Print and shaded views of the part. All mm, measured from the part's lowest x, y and z. A direction names the side the tool comes from. Coordinates: 2 decimals unless noted, no trailing zeros. Order: outer loops, then holes, each group sorted by start corner. A loop starts at its lowest first (then second) coordinate and runs counter-clockwise, first axis right, second up.
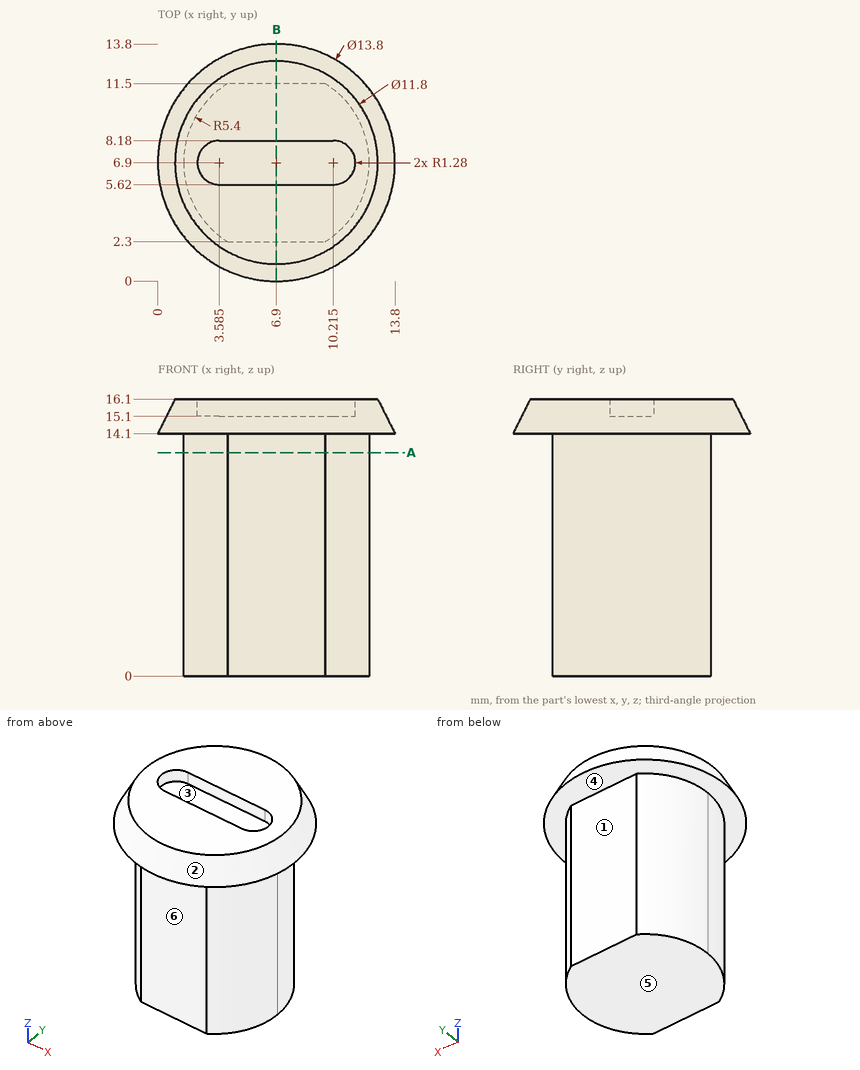
Q1. Drop flat-ended pins along their axis: P1, Ø6, axis at y = 11, z = 10.5, coming from the +X side; P2, Ø1.5, axis at x = 7, z = 3, coming from the +Y side; P3, Ø2, axis at x = 2, z = 2, coming from the -Y side. Give the stop position or say it passes through.
Established:
P1: stops at x = 12.19
P2: stops at y = 11.5
P3: stops at y = 3.17
Q2. Which spindle directions (+Z, -Z, +X, -X, +Y, -Y) get a long thin tool onto all of the face, cutting with end or side? Do the marked faces 4, 5 and 6. Say none if no direction does.
Established:
face 4: -Z
face 5: -Z, +X, -X, +Y, -Y
face 6: -Z, +X, -X, -Y
Q3. Probe line 1 (Z direction, x = 12, y = 4); line 2 (Y direction, x = 5.75, z = 12); line 3 (Z direction, x = 6, y = 8). List the from-to ranges inside material, lowest first.
Established:
line 1: z = 14.1 to 16.1
line 2: y = 2.3 to 11.5
line 3: z = 0 to 15.1
Q4. Cut at A-A, the plane z = 13. List the corners of the cut face in (x, y).
Established:
outline: (1.5, 6.9) arc R5.4 ccw to (4.07, 2.3) - (9.73, 2.3) arc R5.4 ccw to (12.3, 6.9) arc R5.4 ccw to (9.73, 11.5) - (4.07, 11.5) arc R5.4 ccw to start
Q5. Cut at B-B, the plane x = 6.9. List the corners of the cut face in (y, z), plus the area to 3 significant figures.
Established:
outline: (0, 14.1) - (2.3, 14.1) - (2.3, 0) - (11.5, 0) - (11.5, 14.1) - (13.8, 14.1) - (12.8, 16.1) - (8.18, 16.1) - (8.18, 15.1) - (5.62, 15.1) - (5.62, 16.1) - (1, 16.1) - close
area: 153 mm2
Q6. Mould opens along X. For the marked faces 1, 2 and 3 say: pulls with the +X half, pulls with the -X half, needs draft (parallel to the pull), parting line crosses it, or undercut.
Established:
face 1: needs draft
face 2: parting line crosses it
face 3: undercut
